For this review, take the finished solid that the model builds, in its own axes (mm). A direction names the side the tool comes from. Coordinates: 2 decimals unless noted, no trailing zeros. Write each loop counter-clockwise with the first axis right and the second up, starting at its lowest first coordinate (ties: lowest second). Pieces come first, ordered by that corner, then holes.
```python
from build123d import *

# Parameters (mm, degrees)
F0_W     = 146.05
F0_H     = 3.175
F1_DEPTH = 19.05
F2_W     = 73.025
F2_H     = 146.05
F3_DEPTH = 3.175
F4_W     = 7.62
F4_H     = 82.55
F5_DEPTH = 19.05


with BuildPart() as f1:
    # F0 (on Top) → F1 (new body)
    with BuildSketch(Plane.XY):
        Polygon((-73.025, 73.025), (-73.025, 76.2), (-76.2, 76.2), (-76.2, -76.2), (-73.025, -76.2), (-73.025, -73.025), align=None)
        with Locations((0, 74.6125)):
            Rectangle(F0_W, F0_H)
        Polygon((76.2, -76.2), (76.2, 76.2), (73.025, 76.2), (73.025, 73.025), (73.025, -73.025), (73.025, -76.2), align=None)
        with Locations((0, -74.6125)):
            Rectangle(F0_W, F0_H)
    extrude(amount=F1_DEPTH)

    # F2 (on Top) → F3 (join)
    with BuildSketch(Plane.XY):
        with Locations((36.5125, 0)):
            Rectangle(F2_W, F2_H)
    extrude(amount=F3_DEPTH)

    # F4 (on Top) → F5 (join)
    with BuildSketch(Plane.XY):
        with Locations((80.01, 0)):
            Rectangle(F4_W, F4_H)
    extrude(amount=F5_DEPTH)


solid = f1.part
```
Q1. Add section D-D (x = 26.5). State the section outline as (y, z) points (3 decimals), then the cut area to 3 significant figures.
Ans:
outline: (-76.2, 0) - (76.2, 0) - (76.2, 19.05) - (73.025, 19.05) - (73.025, 3.175) - (-73.025, 3.175) - (-73.025, 19.05) - (-76.2, 19.05) - close
area: 585 mm2
Q2. For probe 1 along X at (y, z) = (-29, 6.25) (3 decimals); probe 2 along Y at (x, z) = (32.5, 14.5) (3 decimals), list the stretches that pass through material, from the lowest coordinate up.
Ans:
probe 1: x = -76.2 to -73.025, 73.025 to 83.82
probe 2: y = -76.2 to -73.025, 73.025 to 76.2
Q3. Add section B-B (x = -11). State the section outline as (y, z) points (3 decimals), then the cut area to 3 significant figures.
Ans:
outline: (-76.2, 0) - (-73.025, 0) - (-73.025, 19.05) - (-76.2, 19.05) - close; (73.025, 0) - (76.2, 0) - (76.2, 19.05) - (73.025, 19.05) - close
area: 121 mm2
Q4. Clearance check with flat-ended pins moving along their axes: pin 1 Ø9.5 at (y, z) = (-60.5, 12) entering from +X; pin 2 Ø2.5 at (x, z) = (79, 13) entering from +Y (3 decimals); pin 3 Ø2 at (x, y) = (2, 13.5) entering from +Z (3 decimals). State where each tip first meets the part, or that it passes through.
Ans:
pin 1: stops at x = 76.2
pin 2: stops at y = 41.275
pin 3: stops at z = 3.175
Q5. Tool access review of faces 4 (the flat face through (15, 74, 19.05)), 5 (the flat face through (80, 41.275, 9)), 6 (the flat face through (-73.025, -1, 9)), 7 (the flat face through (73.025, 1, 11)), 8 (the flat face through (76.2, -59, 9)): name each direction out of +Z, -Z, +X, -X, +Y, -Y from which nothing blocks a thin tool from reaching the whole face with its end or side.
Ans:
face 4: +Z, +X, -X, +Y, -Y
face 5: +Z, -Z, +X, +Y
face 6: +Z, -Z
face 7: +Z
face 8: +Z, -Z, +X, -Y
Q6. Draft analysis for pull direction Y (two halves, no side actions). For faces 1 (the flat face through (-1, 73.025, 9)), 2 (the flat face through (80, -41.275, 9)), 3 (the flat face through (83.82, -1, 9)), state which applies: +Y half, -Y half, draft (parallel to the pull), parting line (faces both ways), or undercut.
Ans:
face 1: undercut
face 2: -Y half
face 3: draft
Q7. Add section A-A (y = 32.5). State the section outline as (x, z) points (3 decimals).
Ans:
outline: (-76.2, 0) - (-73.025, 0) - (-73.025, 19.05) - (-76.2, 19.05) - close; (0, 0) - (83.82, 0) - (83.82, 19.05) - (73.025, 19.05) - (73.025, 3.175) - (0, 3.175) - close
Q8. Add section C-C (z = 13.75). State the section outline as (x, y) points (3 decimals), then the cut area to 3 significant figures.
Ans:
outline: (-76.2, -76.2) - (76.2, -76.2) - (76.2, -41.275) - (83.82, -41.275) - (83.82, 41.275) - (76.2, 41.275) - (76.2, 76.2) - (-76.2, 76.2) - close; hole (-73.025, -73.025) - (73.025, -73.025) - (73.025, 73.025) - (-73.025, 73.025) - close
area: 2,520 mm2
